Autodesk Inventor part; units mm, degrees
ref_plane "YZ Plane" through (0, 0, 0) normal (1, 0, 0) x (0, 1, 0)
ref_plane "XZ Plane" through (0, 0, 0) normal (0, 1, 0) x (-1, 0, 0)
ref_plane "XY Plane" through (0, 0, 0) normal (0, 0, 1) x (1, 0, 0)
sketch "Эскиз1" plane through (0, 0, 0) normal (0, 0, 1) x (1, 0, 0)
  circle A0 centre (0, 0) radius 12.5
  dimension "d0" = 25
extrude "Выдавливание1" add sketch "Эскиз1" along normal blind 55.4
sketch "Эскиз2" plane through (0, 0, 55.4) normal (0, 0, 1) x (1, 0, 0)
  circle A0 centre (0, 0) radius 6.75
  dimension "d3" = 13.5
extrude "Выдавливание2" add sketch "Эскиз2" along normal blind 6.55
sketch "Эскиз3" plane through (0, 0, 55.4) normal (0, 0, 1) x (1, 0, 0)
  line L0 (7, 7) -> (13, 7)
  line L1 (13, 7) -> (13, -7)
  line L2 (13, -7) -> (7, -7)
  line L3 (7, -7) -> (7, 7)
  line L4 (-17.6863, 0) -> (18.6175, 0)
  circle A0 centre (0, 0) radius 12.5
  line L5 (-12.5, 0) -> (13, 0)
  point P0 (7, 0)
  dimension "d6" = 6
  dimension "d7" = 14
  dimension "d8" = 25.5
extrude "Выдавливание3" add sketch "Эскиз3" along normal blind 10 contours L0 A0 L4 L3 | L0 L1 L4 A0 | L4 A0 L2 L3 | L4 L1 L2 A0 picked at (8.5105, 3.9415) picked at (8.5105, -3.9415)
sketch "Эскиз4" plane through (0, 0, 0) normal (0, 0, -1) x (-1, 0, 0)
  circle A0 centre (0, 0) radius 3.5
  dimension "d11" = 7
extrude "Выдавливание4" add sketch "Эскиз4" along normal blind 2.7
sketch "Эскиз5" plane through (0, 0, -2.7) normal (0, 0, -1) x (-1, 0, 0)
  circle A0 centre (0, 0) radius 2
  line L0 (1.4283, 1.4) -> (-1.4283, 1.4)
  line L1 (0, -2) -> (0, 1.4)
  dimension "d14" = 4
  dimension "d15" = 3.4
extrude "Выдавливание5" add sketch "Эскиз5" along normal blind 9.7 contours A0 L1 L0 | A0 L0 L1
sketch "Эскиз6" plane through (0, 0, 0) normal (0, 0, -1) x (-1, 0, 0)
  line L0 (0, 8.5) -> (0, -8.5)
  circle A0 centre (0, 8.5) radius 1.5
  circle A1 centre (0, -8.5) radius 1.5
  point P0 (0, 0)
  point P1 (0, 0)
  dimension "d18" = 17
  dimension "d19" = 3
  dimension "d20" = 3
extrude "Выдавливание6" cut sketch "Эскиз6" against normal blind 10
sketch "Эскиз7" plane through (0, 0, 0) normal (0, 1, 0) x (-1, 0, 0)
  line L0 (12.5, 0) -> (-12.5, 0)
  line L1 (12.5, 0) -> (12.5, 22.75)
  line L2 (12.5, 0) -> (12.5, 55.4)
  circle A0 centre (12.5, 22.75) radius 0.5
  line L3 (-2, -12.4) -> (2, -12.4)
  line L4 (0, -12.4) -> (0, 61.95)
  line L5 (6.75, 61.95) -> (-6.75, 61.95)
  point P0 (0, 0)
  point P1 (-1.4283, -12.4)
  point P2 (1.4283, -12.4)
  dimension "d23" = 22.75
  dimension "d24" = 1
revolve "Вращение1" cut sketch "Эскиз7" angle 360 about axis through (0, 0, -12.4) along (0, 0, 1)
properties part number "motor"
Here's how the part is built. I have some questions about the finished solid (model axes, mm). A direction names the side the tool comes from. Coordinates: 2 decimals unless noted, no trailing zeros. Order: outer loops, then holes, each group sorted by start corner. A loop starts at its lowest first (then second) coordinate and runs counter-clockwise, first axis right, second up. Notation, with made-up numbers: (-35, 29.25) - (-28, 29.25) arc R18 cw to (-28, 52.25) - close; hole circle Ø8 at (-15, -33). An arc over 180 degrees is marked (long way). One line per question, with ' | ' between items.
(1) Suppose I cut it at A-A on z = 57. List the corners of the cut face in (x, y) for me, and give its area (3 significant figures).
Report:
outline: circle Ø13.5 at (0, 0); (7, -7) - (13, -7) - (13, 7) - (7, 7) - close | area: 227 mm2
(2) If I drill on L1, parallel to Y at x = 0, z = 6.5; L2, parallel to Z at x = 10.5, y = 4.75; L3, parallel to Z at x = -3.25, y = -8.25, over which ranges is the centre line in solid material (lowest first)?
Report:
L1: y = -12.5 to -10, -7 to 7, 10 to 12.5 | L2: z = 0 to 65.4 | L3: z = 0 to 55.4
(3) Suppose I cut it at B-B on y = 0. List the corners of the cut face in (x, z) for me.
Report:
outline: (-12.5, 0) - (-3.5, 0) - (-3.5, -2.7) - (-2, -2.7) - (-2, -12.4) - (2, -12.4) - (2, -2.7) - (3.5, -2.7) - (3.5, 0) - (12.5, 0) - (12.5, 22.25) arc R0.5 cw to (12.5, 23.25) - (12.5, 55.4) - (13, 55.4) - (13, 65.4) - (7, 65.4) - (7, 55.4) - (6.75, 55.4) - (6.75, 61.95) - (-6.75, 61.95) - (-6.75, 55.4) - (-12.5, 55.4) - (-12.5, 23.25) arc R0.5 cw to (-12.5, 22.25) - close
(4) Suppose I cut it at D-D on z = 2. List the corners of the cut face in (x, y) for me, and give its area (3 significant figures).
Report:
outline: circle Ø25 at (0, 0); hole circle Ø3 at (0, -8.5); hole circle Ø3 at (0, 8.5) | area: 477 mm2
(5) If we mould it in two halves opening along Y, with no side actions, what happens to faces 4 (the cylindrical face through (-3.233, 1.341, -1.331)), 5 (the flat face through (7, 0, 60)), 6 (the flat face through (0, -8, 10))? For each: pulls with the +Y half, pulls with the -Y half, needs draft (parallel to the pull), parting line crosses it, or undercut.
Report:
face 4: parting line crosses it | face 5: needs draft | face 6: undercut
(6) For faces 1 (the flat face through (10, -7, 60)), 2 (the flat face through (0, 9, 10)), 3 (the flat face through (10, 7, 60)), which set-ups out of +Z, -Z, +X, -X, +Y, -Y let a thin tool reach every point of the face, with its end or its side?
Report:
face 1: +Z, +X, -X, -Y | face 2: -Z | face 3: +Z, +X, -X, +Y
(7) Will these pins go through, and if not, where does the flat tip stop? pin 1 (4 mm diameter, centred on y = 3, z = 8.5, fed in from +X); pin 2 (6.5 mm diameter, centred on x = 9, z = 60, fed in from -Y); pin 3 (8 mm diameter, centred on x = 2, y = 8.5, fed in from +Z).
Report:
pin 1: stops at x = 12.46 | pin 2: stops at y = -7 | pin 3: stops at z = 61.95
(8) Suppose I cut it at C-C on x = 0. List the corners of the cut face in (y, z) for me.
Report:
outline: (-12.5, 0) - (-10, 0) - (-10, 10) - (-7, 10) - (-7, 0) - (-3.5, 0) - (-3.5, -2.7) - (-2, -2.7) - (-2, -12.4) - (1.4, -12.4) - (1.4, -2.7) - (3.5, -2.7) - (3.5, 0) - (7, 0) - (7, 10) - (10, 10) - (10, 0) - (12.5, 0) - (12.5, 22.25) arc R0.5 cw to (12.5, 23.25) - (12.5, 55.4) - (6.75, 55.4) - (6.75, 61.95) - (-6.75, 61.95) - (-6.75, 55.4) - (-12.5, 55.4) - (-12.5, 23.25) arc R0.5 cw to (-12.5, 22.25) - close
